Geometry: see drawing. Coordinates: mm, zero at the bounding-box minimum. Coordinates: 2 decimals unless noted, no trailing zeros. One line per item, written item: value. Start each with the question number.
Item 1: Ray query, probe 1 along Y at (x, z) = (1955.8, 979). Return the intervals inside material, ascending. Write a range as from..to.
Item 2: Contact query for flat-ended pins moving along their axis: pin 1 Ø23 at (x, y) = (38.1, 111.125) entering from -Z; pin 2 Ø8 at (x, z) = (1197, 619) entering from -Y. Output: stop coordinate, or through.
Item 3: Section query A-A on z = 1548. Give the number of separate pieces and of enclosed holes in the cut face, then the cut area to 3 significant figures.
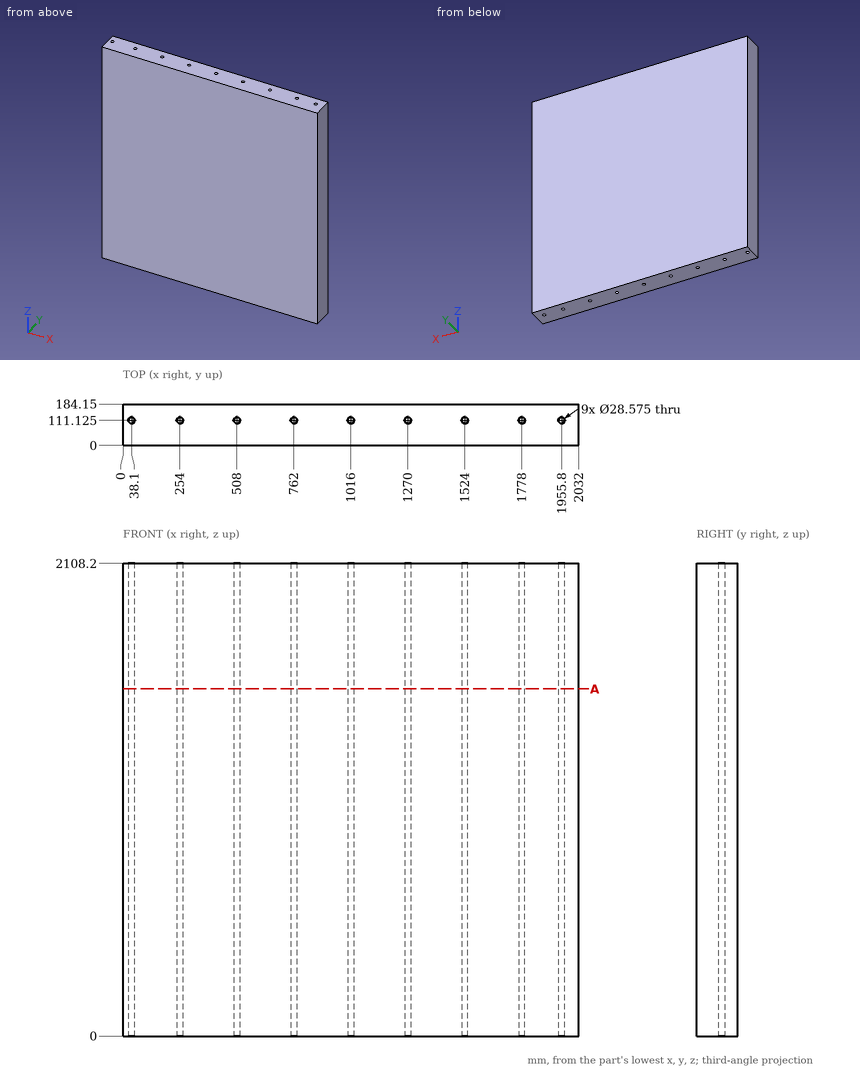
Reply:
1. probe 1: y = 0..96.84, 125.41..184.15
2. pin 1: passes through
2. pin 2: stops at y = 0
3. separate pieces: 1
3. enclosed holes: 9
3. area: 368,000 mm²
